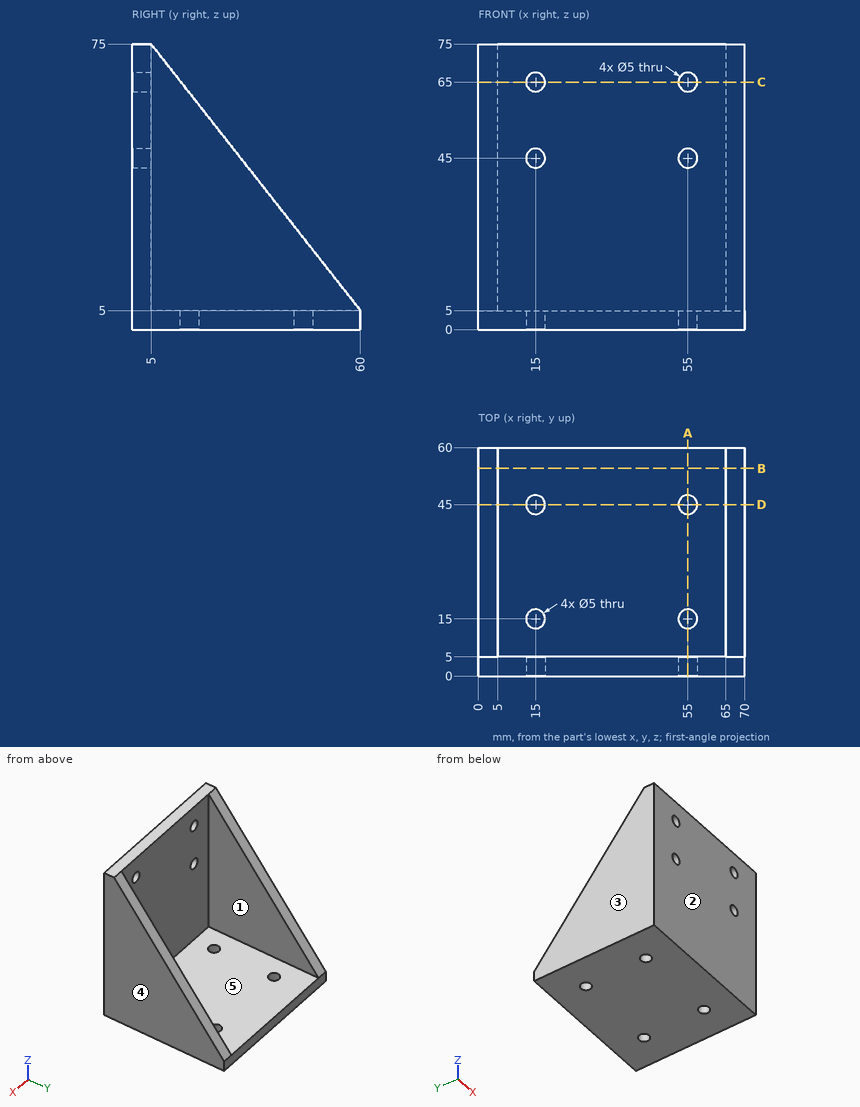
Here's the drawing with two shaded views (mm, measured from the low corner). I have some questions. A direction names the side the tool comes from. Round coordinates to 2 decimals unless told otherwise and drop trailing zeros. Order: outer loops, then holes, each group sorted by start corner. A loop starts at its lowest first (then second) coordinate and runs counter-clockwise, first axis right, second up. Notation, with made-up numbers: (88, 34) -> (110, 34) arc R12 cw to (110, 45) -> close; hole circle Ø3 at (57, -30.75). An arc over 180 degrees is marked (long way). Use a Markdown table: item, result. Add a question column.
(1) For pin 1 Ø6.5 at (x, z) = (15, 65) entering from +Y; pin 2 Ø10 at (x, y) = (19.5, 31) entering from +Z, each with a flat end and sliding along its axis, tell me the tip position at first contact or that it passes through.
(2) For the marked faces 1 and 2, which set-ups out of +Z, -Z, +X, -X, +Y, -Y let a thin tool reach every point of the face, with its end or its side?
(3) Suppose I cut it at C-C, the plane z = 65. Please give me the cut outline in (x, y), and give its area (3 significant figures).
(4) If we mould it in two halves opening along X, with no side actions, what happens to the marked faces 3, 4 and 5? For each: released by +X, released by -X, zero draft, split by the parting line, or undercut.
(5) Suppose I cut it at D-D, the plane y = 45. Please give me the cut outline in (x, z), and give its area (3 significant figures).
(6) I need wall thicknesses on line 1 along Y through (x, z) = (15, 3.8); line 2 along X through (y, z) = (44.5, 20); line 3 along Y through (x, z) = (48.5, 62). Which ranges of each line are inside material? Lowest first, please.
(7) Suppose I cut it at A-A, the plane x = 55. Please give me the cut outline in (y, z).
(8) Suppose I cut it at B-B, the plane y = 54.5. Please give me the cut outline in (x, z), and give its area (3 significant figures).
Verdict:
| question | item | result |
|---|---|---|
| 1 | pin 1 | y = 5 |
| 1 | pin 2 | z = 5 |
| 2 | face 1 | +Z, +Y |
| 2 | face 2 | +Z, -Z, +X, -X, -Y |
| 3 | outline | (0, 0) -> (12.5, 0) -> (12.5, 5) -> (5, 5) -> (5, 12.86) -> (0, 12.86) -> close; (17.5, 0) -> (52.5, 0) -> (52.5, 5) -> (17.5, 5) -> close; (57.5, 0) -> (70, 0) -> (70, 12.86) -> (65, 12.86) -> (65, 5) -> (57.5, 5) -> close |
| 3 | area | 379 mm2 |
| 4 | face 3 | released by -X |
| 4 | face 4 | released by +X |
| 4 | face 5 | undercut |
| 5 | outline | (0, 0) -> (12.5, 0) -> (12.5, 5) -> (5, 5) -> (5, 24.09) -> (0, 24.09) -> close; (17.5, 0) -> (52.5, 0) -> (52.5, 5) -> (17.5, 5) -> close; (57.5, 0) -> (70, 0) -> (70, 24.09) -> (65, 24.09) -> (65, 5) -> (57.5, 5) -> close |
| 5 | area | 491 mm2 |
| 6 | line 1 | 0 to 12.5, 17.5 to 42.5, 47.5 to 60 |
| 6 | line 2 | 0 to 5, 65 to 70 |
| 6 | line 3 | 0 to 5 |
| 7 | outline | (0, 0) -> (12.5, 0) -> (12.5, 5) -> (5, 5) -> (5, 42.5) -> (0, 42.5) -> close; (0, 47.5) -> (5, 47.5) -> (5, 62.5) -> (0, 62.5) -> close; (0, 67.5) -> (5, 67.5) -> (5, 75) -> (0, 75) -> close; (17.5, 0) -> (42.5, 0) -> (42.5, 5) -> (17.5, 5) -> close; (47.5, 0) -> (60, 0) -> (60, 5) -> (47.5, 5) -> close |
| 8 | outline | (0, 0) -> (70, 0) -> (70, 12) -> (65, 12) -> (65, 5) -> (5, 5) -> (5, 12) -> (0, 12) -> close |
| 8 | area | 420 mm2 |
